```python
from build123d import *

# Parameters (mm, degrees)
F_2_56_TAPPED_HOLE1_D           = 1.778
F_2_56_TAPPED_HOLE1_DEPTH       = 3.73
F_2_56_TAPPED_HOLE1_TIP         = 0.53416509
F_4_40_TAPPED_HOLE1_D           = 2.2606
F_4_40_TAPPED_HOLE1_DEPTH       = 7.6
F_4_40_TAPPED_HOLE1_TIP         = 0.679152758
SKETCH_5_R                      = 1.55
CUT_EXTRUDE_1_DEPTH             = 2
CHAMFER_1_SIZE                  = 0.3
CUT_EXTRUDE_2_REACH             = 10.273
SKETCH_6_W                      = 1.2
SKETCH_6_H                      = 1.4
CUT_EXTRUDE_2_DIRECTION_2_REACH = 10.273


with BuildPart() as part:
    # Sketch 1 → Revolve 1 (revolve)
    with BuildSketch(Plane(origin=(0, 0, 0), x_dir=(0, 0, -1), z_dir=(1, 0, 0))):
        Polygon((0, 0), (0, 17), (-3.15, 17), (-3.15, 15.6), (-5.503589838, 15.6), (-5.85, 15), (-5.85, 13), (-5.7, 13), (-5.7, 7.9), (-5.85, 7.9), (-5.85, 5.7), (-5.503589838, 5.1), (-3.65, 5.1), (-3.65, 4.6), (-3.15, 4.6), (-3.15, 4), (-1.25, 4), (-1.25, 3.015093392), (-1.7, 2.7), (-1.7, 0.4), (-1.128740797, 0), align=None)
    revolve(axis=Axis((0, 0, 0), (0, 1, 0)))

    # 2-56 Tapped Hole1
    with Locations(Plane(origin=(0, 10.6, -5.7), x_dir=(-1, 0, 0), z_dir=(0, 0, -1))):
        with Locations((0, 0)):
            Hole(F_2_56_TAPPED_HOLE1_D / 2, depth=F_2_56_TAPPED_HOLE1_DEPTH)
            with Locations((0, 0, -(F_2_56_TAPPED_HOLE1_DEPTH + F_2_56_TAPPED_HOLE1_TIP / 2))):  # 118° drill point
                Cone(0, F_2_56_TAPPED_HOLE1_D / 2, F_2_56_TAPPED_HOLE1_TIP, mode=Mode.SUBTRACT)

    # 4-40 Tapped Hole1
    with Locations(Plane(origin=(0, 17, 0), x_dir=(-1, 0, 0), z_dir=(0, 1, 0))):
        with Locations((0, 0)):
            Hole(F_4_40_TAPPED_HOLE1_D / 2, depth=F_4_40_TAPPED_HOLE1_DEPTH)
            with Locations((0, 0, -(F_4_40_TAPPED_HOLE1_DEPTH + F_4_40_TAPPED_HOLE1_TIP / 2))):  # 118° drill point
                Cone(0, F_4_40_TAPPED_HOLE1_D / 2, F_4_40_TAPPED_HOLE1_TIP, mode=Mode.SUBTRACT)

    # Sketch 5 → Cut-Extrude 1 (cut)
    with BuildSketch(Plane(origin=(0, 17, 0), x_dir=(-1, 0, 0), z_dir=(0, 1, 0))):
        Circle(SKETCH_5_R)
    extrude(amount=-CUT_EXTRUDE_1_DEPTH, mode=Mode.SUBTRACT)

    # Chamfer 1
    chamfer_1_edges = [part.edges().sort_by_distance(p)[0] for p in [
        (1.55, 17, 0),
    ]]
    chamfer(chamfer_1_edges, length=CHAMFER_1_SIZE)

    # Sketch 6 → Cut-Extrude 2 (cut, up to next)
    with BuildSketch(Plane(origin=(0, 0, 0), x_dir=(0.707106781, 0, 0.707106781), z_dir=(-0.707106781, 0, 0.707106781)), mode=Mode.PRIVATE) as cut_extrude_2_sk1:
        with Locations((0, 16.3)):
            Rectangle(SKETCH_6_W, SKETCH_6_H)
    cut_extrude_2_tool1 = extrude(cut_extrude_2_sk1.sketch, amount=-CUT_EXTRUDE_2_REACH, mode=Mode.PRIVATE) & part.part
    add(cut_extrude_2_tool1.solids().sort_by_distance((0, 16.3, 0))[0], mode=Mode.SUBTRACT)

    # Sketch 6 → Cut-Extrude 2 direction 2 (cut, up to next)
    with BuildSketch(Plane(origin=(0, 0, 0), x_dir=(0.707106781, 0, 0.707106781), z_dir=(-0.707106781, 0, 0.707106781)), mode=Mode.PRIVATE) as cut_extrude_2_direction_2_sk1:
        with Locations((0, 16.3)):
            Rectangle(SKETCH_6_W, SKETCH_6_H)
    cut_extrude_2_direction_2_tool1 = extrude(cut_extrude_2_direction_2_sk1.sketch, amount=CUT_EXTRUDE_2_DIRECTION_2_REACH, mode=Mode.PRIVATE) & part.part
    add(cut_extrude_2_direction_2_tool1.solids().sort_by_distance((0, 16.3, 0))[0], mode=Mode.SUBTRACT)


solid = part.part
```
Source: CAD feature listing. Evaluate the final solid. Frame: model axes, mm. A direction names the side the tool comes from. Coordinates: 2 decimals unless noted, no trailing zeros. Loops run counter-clockwise (first coordinate to the right, second up) from the corner with the lowest first, then second, coordinate; pieces in that order, holes last. Notation, with made-up numbers: (71.25, 55) -> (104.25, 55) arc R5 ccw to (104.25, 63) -> close; hole circle Ø11 at (-32.5, -39). An arc over 180 degrees is marked (long way). One line per item, written item: value. Start each with the question number.
Q1. Section query A-A, the plane y = 11.75. Return the cut outline in (x, z).
Q2. Mould query, pull axis Z, two halves, no side actions, for faces 1 (the face through (0, 0, 0)), 2 (the face through (-1.22, 3.5, -0.27)), 3 (the face through (1.156, 16.815, 1.197)). Classes: pulls with the +Z half, pulls with the -Z half, needs draft (parallel to the pull), parting line crosses it, or undercut.
Q3. Section query B-B, the plane y = 7.5. Return the cut outline in (x, z).
Q4. Section query C-C, the plane y = 14.5. Return the cut outline in (x, z), and give its area (3 significant figures).
Q5. Set-up query: faces 4 (the face through (-5.71, 6.78, -1.27)), 5 (the face through (-0.19, 9.73, -3.81)), 6 (the face through (-4, 5.1, 1)), 7 (the face through (-1.166, 16.29, 2.015)). Return all of +Z, -Z, +X, -X, +Y, -Y with unobstructed straight access to the full face (end or side cutting, diameter ignored); none if empty.
Q6. Contact query for flat-ended pins moving along their axis: P1, Ø1, axis at x = -4.5, y = 10.5, coming from the +Z side; P2, Ø4, axis at y = 5.5, z = -3.5, coming from the +X side; P3, Ø4, axis at y = 9.5, z = 4, coming from the +X side. Output: stop coordinate, or through.
Q7. Line query: line 1 along X through (y, z) = (11.9, 0); line 2 along Z through (x, y) = (0, 16.4); line 3 along Y through (x, z) = (-3.5, 0.5). Output: solid intervals per line, ascending.
Results:
1. outline: circle Ø11.4 at (0, 0); hole circle Ø2.26 at (0, 0)
2. face 1: needs draft
2. face 2: parting line crosses it
2. face 3: undercut
3. outline: circle Ø11.7 at (0, 0)
4. outline: circle Ø11.7 at (0, 0); hole circle Ø2.26 at (0, 0)
4. area: 103 mm^2
5. face 4: +Y, -Y
5. face 5: -Z
5. face 6: -Y
5. face 7: +Y
6. P1: z = 4.06
6. P2: x = 5.65
6. P3: x = 5.34
7. line 1: -5.7 to -1.13, 1.13 to 5.7
7. line 2: -3.15 to -1.55, 1.55 to 3.15
7. line 3: 4.6 to 15.6
